from build123d import *

# Parameters (mm, degrees)
BOSS_EXTRUDE1_DEPTH = 3


with BuildPart() as part:
    # Sketch1 → Boss-Extrude1 (new body)
    with BuildSketch(Plane(origin=(0, 0, 0), x_dir=(1, 0, 0), z_dir=(0, 1, 0))):
        Polygon((-9.419602878, 89.5), (-8, 64.5), (0, 64.5), (0, 89.5), align=None)
    boss_extrude1 = extrude(amount=BOSS_EXTRUDE1_DEPTH)

    # Mirror1: Boss-Extrude1 across plane
    add(boss_extrude1.mirror(Plane(origin=(0, 0, 0), x_dir=(0, 0, 1), z_dir=(1, 0, 0))))

    # Sketch2 → Cut-Revolve1 (revolve, cut)
    with BuildSketch(Plane(origin=(0, 0, 0), x_dir=(0, 0, -1), z_dir=(1, 0, 0))):
        with BuildLine():
            Line((72.5, 6), (77.5, 6))
            Line((77.5, 6), (77.5, 1))
            ThreePointArc((77.5, 1), (73.964466094, 2.464466094), (72.5, 6))
        make_face()
    revolve(axis=Axis((0, 6, -77.5), (0, -1, 0)), mode=Mode.SUBTRACT)


solid = part.part
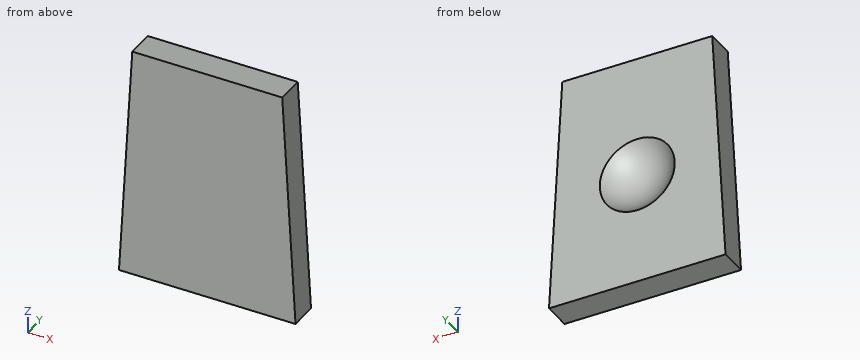
Check sheet for the modelled part. Datum: model origin and axes. Units: mm. Round coordinates to 2 decimals unless told otherwise and drop trailing zeros. Loops run counter-clockwise (first coordinate to the right, second up) from the corner with the lowest first, then second, coordinate; pieces in that order, holes last.
1. Gauge pin test, flat ends, axial feed: pin 1 Ø1 at (y, z) = (2, -73) entering from -X; pin 2 Ø8 at (x, z) = (-2.5, -78) entering from +Y. Record the tip position at first contact, or that the pin passes through.
2. Sectioned sample at A-A on y = 2.65. Record the boundary of the cut face in (x, z).
3. Sectioned sample at B-B on z = -76. Record the boundary of the cut face in (x, y), and give its area (3 significant figures).
4. Sectioned sample at D-D on y = 0.3. Record the boundary of the cut face in (x, z).
5. Sectioned sample at C-C on x = 3. Record the boundary of the cut face in (y, z), and give its area (3 significant figures).
6. Scan lines: probe 1 along X at (y, z) = (2.9, -80); probe 2 along Z at (x, y) = (1.75, 2.15); probe 3 along Z at (x, y) = (-1.25, 2.3). Record each from-to range of solid material in increasing order.
Recorded:
1. pin 1: stops at x = -8.51
1. pin 2: stops at y = 3
2. outline: (-9.42, -89.5) - (9.42, -89.5) - (8, -64.5) - (-8, -64.5) - close; hole circle Ø7.42 at (0, -77.5)
3. outline: (-8.65, 0) - (8.65, 0) - (8.65, 3) - (3.71, 3) arc R4.77 cw to (-3.71, 3) - (-8.65, 3) - close
3. area: 42.8 mm2
4. outline: (-9.42, -89.5) - (9.42, -89.5) - (8, -64.5) - (-8, -64.5) - close
5. outline: (0, -89.5) - (3, -89.5) - (3, -80.15) arc R4 cw to (3, -74.85) - (3, -64.5) - (0, -64.5) - close
5. area: 71.4 mm2
6. probe 1: x = -8.88 to -3.02, 3.02 to 8.88
6. probe 2: z = -89.5 to -80.17, -74.83 to -64.5
6. probe 3: z = -89.5 to -80.62, -74.38 to -64.5
